Check sheet for the modelled part. Datum: model origin and axes. Units: mm. Round coordinates to 2 decimals unless told otherwise and drop trailing zeros. Order: outer loops, then holes, each group sorted by start corner. A loop starts at its lowest first (then second) coordinate and runs counter-clockwise, first axis right, second up. Notation, with made-up numbers: (-26.75, 29.25) -> (3.25, 29.25) arc R11 ccw to (3.25, 37.25) -> close; hole circle Ø1 at (-24.5, 60.25). An arc over 180 degrees is marked (long way). Answer in a Markdown table with one row per item.
from build123d import *

# Parameters (mm, degrees)
F0_R     = 11
F1_DEPTH = 3


with BuildPart() as f1:
    # F0 (on Top) → F1 (new body)
    with BuildSketch(Plane.XY):
        with BuildLine():
            ThreePointArc((-27.625907, -38.023799), (-5.725919, -36.403446), (-3.695413, -14.537673))
            ThreePointArc((-3.695413, -14.537673), (0, -15), (3.695413, -14.537673))
            ThreePointArc((3.695413, -14.537673), (5.725919, -36.403446), (27.625907, -38.023799))
            ThreePointArc((27.625907, -38.023799), (32.852328, -16.694956), (12.684203, -8.006934))
            ThreePointArc((12.684203, -8.006934), (14.265848, -4.635255), (14.968094, -0.977841))
            ThreePointArc((14.968094, -0.977841), (44.699656, 14.523799), (11.534681, 9.589115))
            ThreePointArc((11.534681, 9.589115), (8.816779, 12.135255), (5.555378, 13.933333))
            ThreePointArc((5.555378, 13.933333), (0, 47), (-5.555378, 13.933333))
            ThreePointArc((-5.555378, 13.933333), (-8.816779, 12.135255), (-11.534681, 9.589115))
            ThreePointArc((-11.534681, 9.589115), (-44.699656, 14.523799), (-14.968094, -0.977841))
            ThreePointArc((-14.968094, -0.977841), (-14.265848, -4.635255), (-12.684203, -8.006934))
            ThreePointArc((-12.684203, -8.006934), (-32.852328, -16.694956), (-27.625907, -38.023799))
        make_face()
        with Locations((-17.633558, -24.27051)):
            Circle(F0_R, mode=Mode.SUBTRACT)
        Circle(F0_R, mode=Mode.SUBTRACT)
        with Locations((17.633558, -24.27051)):
            Circle(F0_R, mode=Mode.SUBTRACT)
        with Locations((-28.531695, 9.27051)):
            Circle(F0_R, mode=Mode.SUBTRACT)
        with Locations((0, 30)):
            Circle(F0_R, mode=Mode.SUBTRACT)
        with Locations((28.531695, 9.27051)):
            Circle(F0_R, mode=Mode.SUBTRACT)
    extrude(amount=F1_DEPTH)


solid = f1.part
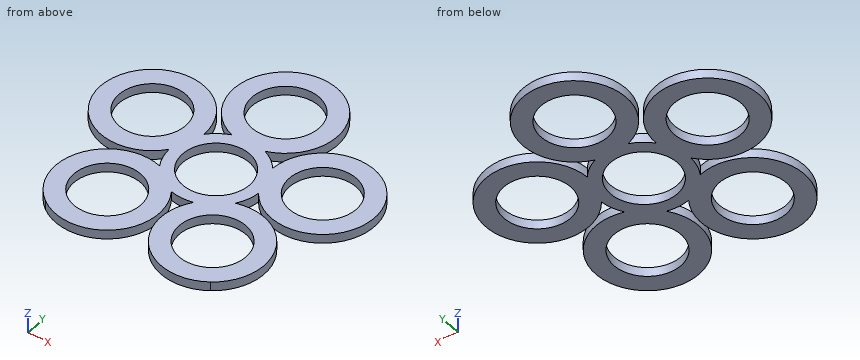
Item 1: Cross-section at A-A (y = 30). Record the boundary of the cut face in (x, z), and give its area (3 significant figures).
Result sheet:
| item | result |
|---|---|
| outline | (-17, 0) -> (-11, 0) -> (-11, 3) -> (-17, 3) -> close; (11, 0) -> (17, 0) -> (17, 3) -> (11, 3) -> close |
| area | 36.0 mm^2 |
Item 2: Cross-section at B-B (x = 24.5). Record the boundary of the cut face in (y, z), and give its area (3 significant figures).
Result sheet:
| item | result |
|---|---|
| outline | (-39.82, 0) -> (-32.86, 0) -> (-32.86, 3) -> (-39.82, 3) -> close; (-15.68, 0) -> (-8.72, 0) -> (-8.72, 3) -> (-15.68, 3) -> close; (-7.24, 0) -> (-0.96, 0) -> (-0.96, 3) -> (-7.24, 3) -> close; (19.51, 0) -> (25.79, 0) -> (25.79, 3) -> (19.51, 3) -> close |
| area | 79.4 mm^2 |
Item 3: Cross-section at C-C (y = -6). Record the boundary of the cut face in (x, z), and give its area (3 significant figures).
Result sheet:
| item | result |
|---|---|
| outline | (-36, 0) -> (-21.06, 0) -> (-21.06, 3) -> (-36, 3) -> close; (-13.75, 0) -> (-9.22, 0) -> (-9.22, 3) -> (-13.75, 3) -> close; (9.22, 0) -> (13.75, 0) -> (13.75, 3) -> (9.22, 3) -> close; (21.06, 0) -> (36, 0) -> (36, 3) -> (21.06, 3) -> close |
| area | 117 mm^2 |
Item 4: Scan lines: line 1 (X direction, y = 15, z = 0.6); line 2 (Y direction, x = 6, z = 1.7); line 3 (X direction, y = -21, z = 2.6). Record each from-to range of solid material in increasing order. Write a range as [from, to].
Result sheet:
| item | result |
|---|---|
| line 1 | x = [-44.54, -37.92], [-19.14, -12.53], [-8, 8], [12.53, 19.14], [37.92, 44.54] |
| line 2 | y = [-36.67, -9.22], [9.22, 13.75], [14.09, 20.78], [39.22, 45.91] |
| line 3 | x = [-34.32, -28.14], [-7.13, -0.95], [0.95, 7.13], [28.14, 34.32] |
Item 5: Cross-section at D-D (z = 1.35). Record the boundary of the cut face in (x, y), and give its area (3 significant figures).
Result sheet:
| item | result |
|---|---|
| outline | (-14.97, -0.98) arc R15 ccw to (-12.68, -8.01) arc R17 ccw (long way) to (-3.7, -14.54) arc R15 ccw to (3.7, -14.54) arc R17 ccw (long way) to (12.68, -8.01) arc R15 ccw to (14.97, -0.98) arc R17 ccw (long way) to (11.53, 9.59) arc R15 ccw to (5.56, 13.93) arc R17 ccw (long way) to (-5.56, 13.93) arc R15 ccw to (-11.53, 9.59) arc R17 ccw (long way) to start; hole circle Ø22 at (-28.53, 9.27); hole circle Ø22 at (-17.63, -24.27); hole circle Ø22 at (0, 0); hole circle Ø22 at (0, 30); hole circle Ø22 at (17.63, -24.27); hole circle Ø22 at (28.53, 9.27) |
| area | 2,890 mm^2 |
Item 6: Depth check by flat-ended pin: P1, Ø1, axis at y = -30, z = 1, coming from the +X side; P2, Ø1.5, axis at y = -10.5, z = 1, coming from the +X side. Enter the tip coordinate at first touch or a pass-through.
Result sheet:
| item | result |
|---|---|
| P1 | stops at x = 33.81 |
| P2 | stops at x = 28.56 |
